Part model, mm, in its own coordinate system. Give positions to 0.01 mm unless a question says otherwise; leave off trailing zeros. Loops run counter-clockwise (first coordinate to the right, second up) from the corner with the lowest first, then second, coordinate; pieces in that order, holes last. Notation, with made-up numbers: M -14.5,42 L -10.5,42 A20 cw -10.5,57 Z; hole C 59,53.5 d9. An arc over 180 degrees is marked long. Answer in a Markdown table with one row per item.
from build123d import *

# Parameters (mm, degrees)
IZIM1_W                     = 79.8
IZIM1_H                     = 70
Y_KSEKLIK_EKSTR_ZYON1_DEPTH = 4
RADYUS1_R                   = 5
RADYUS2_R                   = 5
DELIK1_D                    = 4.2
DELIK1_DEPTH                = 5
DELIK1_CSINK_D              = 6.5
DELIK1_CSINK_ANGLE          = 80


with BuildPart() as part:
    # Çizim1 → Yükseklik-Ekstrüzyon1 (new body)
    with BuildSketch(Plane.XY):
        Rectangle(IZIM1_W, IZIM1_H)
    extrude(amount=Y_KSEKLIK_EKSTR_ZYON1_DEPTH)

    # Radyus1
    radyus1_edges = [part.edges().sort_by_distance(p)[0] for p in [
        (39.9, -35, 2),
        (-39.9, -35, 2),
        (-39.9, 35, 2),
        (39.9, 35, 2),
    ]]
    fillet(radyus1_edges, radius=RADYUS1_R)

    # Radyus2
    # the kernel refuses this fillet: 5 mm, written as the material it takes off along each edge
    with BuildSketch(Plane(origin=(34.9, -30, 0), x_dir=(0, -1, 0), z_dir=(-1, 0, 0))) as radyus2_piece_1:
        with BuildLine():
            CenterArc((0.101020514, 5), RADYUS2_R, 270, 78.463040967)
            Line((5, 4), (5.09797959, 3.98))
            ThreePointArc((5.09797959, 3.98), (5.1, 2), (5.1, 0))
            Line((5.1, 0), (5, -0.1))
            Line((5, -0.1), (0.101020514, -0.1))
            Line((0.101020514, -0.1), (0.101020514, 0))
        make_face()
    revolve(axis=Axis((34.9, -30, 0), (0, 0, 1)), revolution_arc=90, mode=Mode.SUBTRACT)
    with BuildSketch(Plane(origin=(-34.9, -35, 0), x_dir=(0, 1.5720758028687172e-12, 1.0), z_dir=(1, 0, 0))) as radyus2_piece_2:
        with BuildLine():
            CenterArc((5, -4.898979486), RADYUS2_R, 101.536959033, 78.463040967)
            Line((0, -4.898979486), (-0.1, -4.898979486))
            Line((-0.1, -4.898979486), (-0.1, 0))
            Line((-0.1, 0), (0, 0.1))
            ThreePointArc((0, 0.1), (2, 0.1), (3.98, 0.09797959))
            Line((3.98, 0.09797959), (4, 0))
        make_face()
    extrude(amount=69.8, mode=Mode.SUBTRACT)
    with BuildSketch(Plane(origin=(-34.9, -30, 0), x_dir=(0, -1, 0), z_dir=(1, 0, 0))) as radyus2_piece_3:
        with BuildLine():
            CenterArc((0.101020514, -5), RADYUS2_R, 11.536959033, 78.463040967)
            Line((5, -4), (5.09797959, -3.98))
            ThreePointArc((5.09797959, -3.98), (5.1, -2), (5.1, 0))
            Line((5.1, 0), (5, 0.1))
            Line((5, 0.1), (0.101020514, 0.1))
            Line((0.101020514, 0.1), (0.101020514, 0))
        make_face()
    revolve(axis=Axis((-34.9, -30, 0), (0, 0, -1)), revolution_arc=90, mode=Mode.SUBTRACT)
    with BuildSketch(Plane(origin=(-39.9, 30, 0), x_dir=(1, 0, 0), z_dir=(0, -1, 0)), Plane(origin=(39.9, -30, 0), x_dir=(-1, 0, 0), z_dir=(0, 1, 0))) as radyus2_piece_4:
        with BuildLine():
            CenterArc((4.898979486, 5), RADYUS2_R, 191.536959033, 78.463040967)
            Line((0, 4), (-0.09797959, 3.98))
            ThreePointArc((-0.09797959, 3.98), (-0.1, 2), (-0.1, 0))
            Line((-0.1, 0), (0, -0.1))
            Line((0, -0.1), (4.898979486, -0.1))
            Line((4.898979486, -0.1), (4.898979486, 0))
        make_face()
    extrude(amount=60, mode=Mode.SUBTRACT)
    with BuildSketch(Plane(origin=(-34.9, 30, 0), x_dir=(0, 1, 0), z_dir=(1, 0, 0))) as radyus2_piece_5:
        with BuildLine():
            CenterArc((0.101020514, 5), RADYUS2_R, 270, 78.463040967)
            Line((5, 4), (5.09797959, 3.98))
            ThreePointArc((5.09797959, 3.98), (5.1, 2), (5.1, 0))
            Line((5.1, 0), (5, -0.1))
            Line((5, -0.1), (0.101020514, -0.1))
            Line((0.101020514, -0.1), (0.101020514, 0))
        make_face()
    revolve(axis=Axis((-34.9, 30, 0), (0, 0, 1)), revolution_arc=90, mode=Mode.SUBTRACT)
    with BuildSketch(Plane(origin=(34.9, 35, 0), x_dir=(0, -1, 0), z_dir=(-1, 0, 0))) as radyus2_piece_6:
        with BuildLine():
            CenterArc((4.898979486, 5), RADYUS2_R, 191.536959033, 78.463040967)
            Line((0, 4), (-0.09797959, 3.98))
            ThreePointArc((-0.09797959, 3.98), (-0.1, 2), (-0.1, 0))
            Line((-0.1, 0), (0, -0.1))
            Line((0, -0.1), (4.898979486, -0.1))
            Line((4.898979486, -0.1), (4.898979486, 0))
        make_face()
    extrude(amount=69.8, mode=Mode.SUBTRACT)
    with BuildSketch(Plane(origin=(34.9, 30, 0), x_dir=(1, 0, 0), z_dir=(0, -1, 0))) as radyus2_piece_7:
        with BuildLine():
            CenterArc((0.101020514, 5), RADYUS2_R, 270, 78.463040967)
            Line((5, 4), (5.09797959, 3.98))
            ThreePointArc((5.09797959, 3.98), (5.1, 2), (5.1, 0))
            Line((5.1, 0), (5, -0.1))
            Line((5, -0.1), (0.101020514, -0.1))
            Line((0.101020514, -0.1), (0.101020514, 0))
        make_face()
    revolve(axis=Axis((34.9, 30, 0), (0, 0, 1)), revolution_arc=90, mode=Mode.SUBTRACT)

    # Delik1
    with Locations(Plane(origin=(0, 0, 0), x_dir=(-1, 0, 0), z_dir=(0, 0, -1))):
        with Locations((-35.667766953, 30.767766953), (35.667766953, 30.767766953), (35.667766953, -30.767766953), (-35.667766953, -30.767766953)):
            CounterSinkHole(DELIK1_D / 2, DELIK1_CSINK_D / 2, depth=DELIK1_DEPTH, counter_sink_angle=DELIK1_CSINK_ANGLE)


solid = part.part
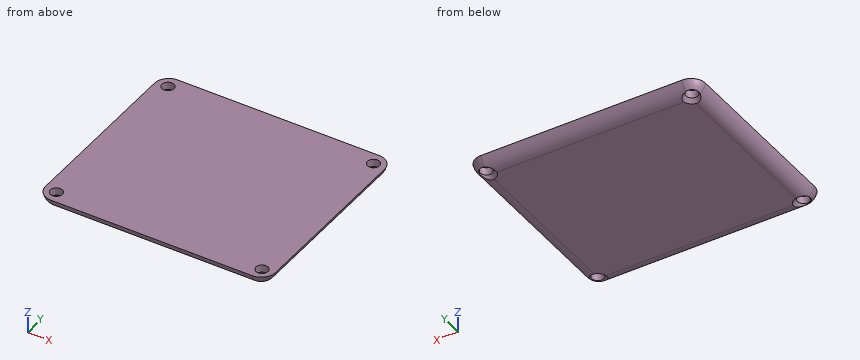
(1) Pin check, flat tips, straight feed: pin 1 Ø2 at (x, z) = (26.5, 1) entering from -Y; pin 2 Ø2 at (x, z) = (0, 2) entering from -Y; pin 3 Ø1.5 at (y, z) = (-9, 1.5) entering from -X. Stop position of each tip, or through.
Recorded:
| item | result |
|---|---|
| pin 1 | stops at y = -34.1 |
| pin 2 | stops at y = -34.68 |
| pin 3 | stops at x = -39.18 |
(2) Saw through at B-B (x = 0.5). Write the cut outline in (y, z), plus the area to 3 significant figures.
Recorded:
| item | result |
|---|---|
| outline | M -35,4 A5 ccw -30.1,0 L 30.1,0 A5 ccw 35,4 Z |
| area | 270 mm^2 |
(3) Saw through at C-C (z = 2.1). Give the number of separate pieces and of enclosed holes in the cut face, plus the area to 3 significant figures.
Recorded:
| item | result |
|---|---|
| separate pieces | 1 |
| enclosed holes | 4 |
| area | 5,270 mm^2 |
(4) Saw through at A-A (y = 11). Write the cut outline in (x, z).
Recorded:
| item | result |
|---|---|
| outline | M -39.9,4 A5 ccw -35,0 L 35,0 A5 ccw 39.9,4 Z |
(5) Drill centre lines: line 1 along Y through (x, z) = (-14, 3.8); line 2 along X through (y, z) = (-23, 3.7); line 3 along Y through (x, z) = (5.5, 3.5). Where is each one in solid material? Low to high.
Recorded:
| item | result |
|---|---|
| line 1 | y = -34.95 to 34.95 |
| line 2 | x = -39.83 to 39.83 |
| line 3 | y = -34.87 to 34.87 |
